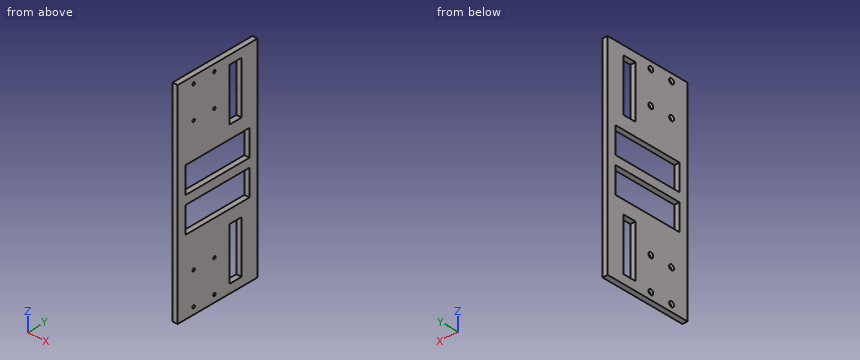
```python
from build123d import *

# Parameters (mm, degrees)
SKETCH_1_W          = 240
SKETCH_1_H          = 100
EXTRUDE_1_DEPTH     = 6
SKETCH_2_R          = 1.55
CUT_EXTRUDE_1_DEPTH = 261.069221555
SKETCH_3_W          = 60
SKETCH_3_H          = 15
CUT_EXTRUDE_2_DEPTH = 261.069221555
SKETCH_4_W          = 30
SKETCH_4_H          = 80
CUT_EXTRUDE_3_DEPTH = 261.069221555
SKETCH_5_R          = 3
CUT_EXTRUDE_4_DEPTH = 3


with BuildPart() as part:
    # 草图1 → 凸台-拉伸1 (new body)
    with BuildSketch(Plane(origin=(0, 0, 0), x_dir=(0, 0, -1), z_dir=(1, 0, 0))):
        with Locations((120, -50)):
            Rectangle(SKETCH_1_W, SKETCH_1_H)
    extrude(amount=EXTRUDE_1_DEPTH)

    # 草图2 → 切除-拉伸1 (cut, through all)
    with BuildSketch(Plane(origin=(6, 0, 0), x_dir=(0, 0, -1), z_dir=(1, 0, 0))):
        with Locations((8, -54)):
            Circle(SKETCH_2_R)
        with Locations((45, -80)):
            Circle(SKETCH_2_R)
        with Locations((45, -54)):
            Circle(SKETCH_2_R)
        with Locations((8, -80)):
            Circle(SKETCH_2_R)
        with Locations(Location((232, -80, 0), (0, 0, 180))):
            Circle(SKETCH_2_R)
        with Locations(Location((195, -54, 0), (0, 0, 180))):
            Circle(SKETCH_2_R)
        with Locations(Location((195, -80, 0), (0, 0, 180))):
            Circle(SKETCH_2_R)
        with Locations(Location((232, -54, 0), (0, 0, 180))):
            Circle(SKETCH_2_R)
    extrude(amount=-CUT_EXTRUDE_1_DEPTH, mode=Mode.SUBTRACT)

    # 草图3 → 切除-拉伸2 (cut, through all)
    with BuildSketch(Plane(origin=(6, 0, 0), x_dir=(0, 0, -1), z_dir=(1, 0, 0))):
        with Locations((40, -27.5)):
            Rectangle(SKETCH_3_W, SKETCH_3_H)
        with Locations((200, -27.5)):
            Rectangle(SKETCH_3_W, SKETCH_3_H)
    extrude(amount=-CUT_EXTRUDE_2_DEPTH, mode=Mode.SUBTRACT)

    # 草图4 → 切除-拉伸3 (cut, through all)
    with BuildSketch(Plane(origin=(6, 0, 0), x_dir=(0, 0, -1), z_dir=(1, 0, 0))):
        with Locations((100, -50)):
            Rectangle(SKETCH_4_W, SKETCH_4_H)
        with Locations((140, -50)):
            Rectangle(SKETCH_4_W, SKETCH_4_H)
    extrude(amount=-CUT_EXTRUDE_3_DEPTH, mode=Mode.SUBTRACT)

    # 草图5 → 切除-拉伸4 (cut)
    with BuildSketch(Plane.ZY):
        with Locations((-195, -80)):
            Circle(SKETCH_5_R)
        with Locations((-232, -80)):
            Circle(SKETCH_5_R)
        with Locations((-195, -54)):
            Circle(SKETCH_5_R)
        with Locations((-232, -54)):
            Circle(SKETCH_5_R)
        with Locations((-45, -80)):
            Circle(SKETCH_5_R)
        with Locations((-8, -80)):
            Circle(SKETCH_5_R)
        with Locations((-8, -54)):
            Circle(SKETCH_5_R)
        with Locations((-45, -54)):
            Circle(SKETCH_5_R)
    extrude(amount=-CUT_EXTRUDE_4_DEPTH, mode=Mode.SUBTRACT)


solid = part.part
```
The listing builds one solid part. Answer for the finished solid, in the listing's coordinates (mm). Coordinates: 2 decimals unless noted, no trailing zeros. Loops run counter-clockwise (first coordinate to the right, second up) from the corner with the lowest first, then second, coordinate; pieces in that order, holes last. Notation, with made-up numbers: M 49.5,44 L 87.5,44 A34 ccw 87.5,75 Z; hole C -38,6.25 d9. An arc over 180 degrees is marked long. Answer as a JSON object with one key per item and string values. Group by question number.
Item 1: Each of these flat-tipped pins is pushed along its axis until it touches: P1, Ø1.9, axis at y = -54, z = -8, coming from the +X side; P2, Ø5, axis at y = -80, z = -45, coming from the -X side. Where does it stop, or does it pass through?
Item 2: Consider L1, parallel to Y at x = 1.35, z = -232; L2, parallel to Z at x = 3.85, y = -42; L3, parallel to Y at x = 1.85, z = -195. Determine where each line is inside the solid, lowest interval first.
Item 3: Section D-D (z = -94) is taken. Write down the section's boundary in (x, y), and give its area (3 significant figures).
Item 4: Section A-A (z = -187.5) is taken. Write down the section's boundary in (x, y), and give its area (3 significant figures).
Item 5: Section B-B (y = -43) is taken. Write down the section's boundary in (x, z).
Item 6: Section C-C (x = 2) is taken. Give the number of separate pieces and of enclosed holes in the cut face, and give its area (3 significant figures).
Solved:
{
 "1": {"P1": "passes through", "P2": "stops at x = 3"},
 "2": {"L1": "y = -100 to -83, -77 to -57, -51 to 0", "L2": "z = -240 to -155, -125 to -115, -85 to 0", "L3": "y = -100 to -83, -77 to -57, -51 to -35, -20 to 0"},
 "3": {"outline": "M 0,-100 L 6,-100 L 6,-90 L 0,-90 Z; M 0,-10 L 6,-10 L 6,0 L 0,0 Z", "area": "120 mm2"},
 "4": {"outline": "M 0,-100 L 6,-100 L 6,-35 L 0,-35 Z; M 0,-20 L 6,-20 L 6,0 L 0,0 Z", "area": "510 mm2"},
 "5": {"outline": "M 0,-240 L 6,-240 L 6,-155 L 0,-155 Z; M 0,-125 L 6,-125 L 6,-115 L 0,-115 Z; M 0,-85 L 6,-85 L 6,0 L 0,0 Z"},
 "6": {"separate pieces": "1", "enclosed holes": "12", "area": "17,200 mm2"}
}
